```python
from build123d import *

# Parameters (mm, degrees)
EXTRUDE_1_DEPTH        = 3
HOLE_WIZARD_M4_1_D     = 4.5
HOLE_WIZARD_M4_1_DEPTH = 20
HOLE_WIZARD_M4_1_TIP   = 1.351936393


with BuildPart() as part:
    # ｽｹｯﾁ1 → ﾎﾞｽ - 押し出し1 (new body)
    with BuildSketch(Plane.XY):
        Polygon((3.954849344, 0), (1.977424672, 3.425), (-1.977424672, 3.425), (-3.954849344, 0), (-1.977424672, -3.425), (1.977424672, -3.425), align=None)
    extrude(amount=EXTRUDE_1_DEPTH)

    # M4 すきま穴1
    with Locations(Plane.XY.offset(3)):
        with Locations((0, 0)):
            Hole(HOLE_WIZARD_M4_1_D / 2, depth=HOLE_WIZARD_M4_1_DEPTH)
            with Locations((0, 0, -(HOLE_WIZARD_M4_1_DEPTH + HOLE_WIZARD_M4_1_TIP / 2))):  # 118° drill point
                Cone(0, HOLE_WIZARD_M4_1_D / 2, HOLE_WIZARD_M4_1_TIP, mode=Mode.SUBTRACT)


solid = part.part
```
The model under review builds one solid part; all positions refer to its coordinate system, in mm. Give positions to 0.01 mm unless a question says otherwise; leave off trailing zeros. Write each loop counter-clockwise with the first axis right and the second up, starting at its lowest first coordinate (ties: lowest second). Pieces come first, ordered by that corner, then holes.
(1) The part is to be moulded in two halves that separate along Y. For faces 1 (the flat face through (0, 3.425, 1)), 2 (the flat face through (2.95, -1.74, 1.48)), 3 (the cylindrical face through (0.29, 2.23, 1.48)), say which applies: released by +Y, released by -Y, zero draft, split by the parting line, or undercut.
(2) Consider section A-A, the plane x = 0.25. Give the boundary of the cut face in (y, z) (3 decimals), and give its area (3 significant figures).
(3) Consider section B-B, the plane z = 1.4. Give the boundary of the cut face in (x, y) (3 decimals), and give its area (3 significant figures).
(4) To check wall thickness, follow L1, parallel to Y at x = 0, z = 1.35 (3 decimals); L2, parallel to X at y = -1, z = 1.25; L3, parallel to Y at x = -0.75, z = 2.1 (3 decimals). State the ranges of each line that lie inside material, in increasing order.
(5) Consider section D-D, the plane x = -2.75. Give the boundary of the cut face in (y, z).
(6) Consider section C-C, the plane y = -1. Give the boundary of the cut face in (x, z), and give its area (3 significant figures).
Returned:
1. face 1: released by +Y
1. face 2: released by -Y
1. face 3: undercut
2. outline: (-3.425, 0) - (-2.236, 0) - (-2.236, 3) - (-3.425, 3) - close; (2.236, 0) - (3.425, 0) - (3.425, 3) - (2.236, 3) - close
2. area: 7.13 mm2
3. outline: (-3.955, 0) - (-1.977, -3.425) - (1.977, -3.425) - (3.955, 0) - (1.977, 3.425) - (-1.977, 3.425) - close; hole circle Ø4.5 at (0, 0)
3. area: 24.7 mm2
4. L1: y = -3.425 to -2.25, 2.25 to 3.425
4. L2: x = -3.38 to -2.02, 2.02 to 3.38
4. L3: y = -3.425 to -2.121, 2.121 to 3.425
5. outline: (-2.09, 0) - (2.09, 0) - (2.09, 3) - (-2.09, 3) - close
6. outline: (-3.38, 0) - (-2.02, 0) - (-2.02, 3) - (-3.38, 3) - close; (2.02, 0) - (3.38, 0) - (3.38, 3) - (2.02, 3) - close
6. area: 8.17 mm2
